Geometry: see drawing. Coordinates: mm, zero at the bounding-box minimum. A direction names the side the tool comes from. Round coordinates to 2 decimals unless told otherwise and drop trailing zeros. Loops run counter-clockwise (first coordinate to the right, second up) from the corner with the lowest first, then second, coordinate; pieces in that order, holes last. Notation, with made-up numbers: (-35.5, 45.5) -> (8.5, 45.5) arc R16 cw to (8.5, 74.5) -> close; hole circle Ø9 at (89, -28.5). An arc over 180 degrees is marked (long way). Write item = value, one per line.
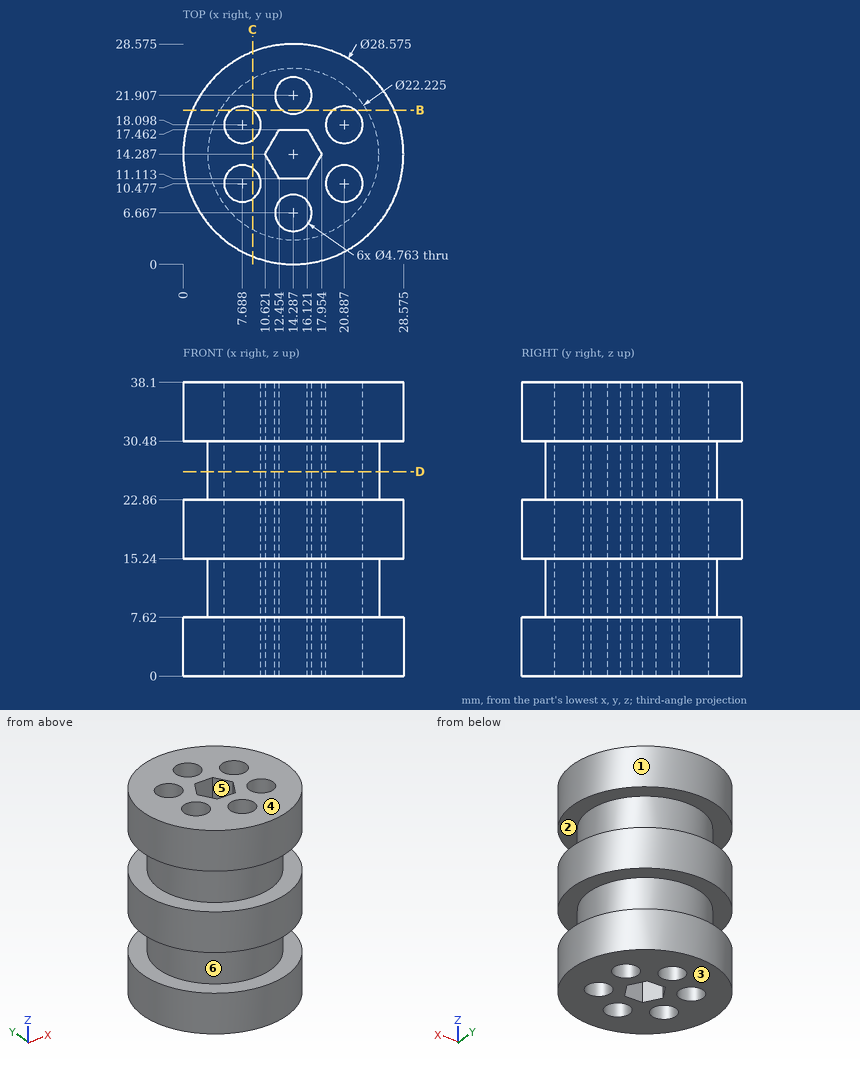
1. Line query: probe 1 along Z at (x, y) = (8.25, 24); probe 2 along Y at (x, z) = (14.25, 18) (1 decimal); probe 3 along X at (y, z) = (8.5, 14) (1 decimal). Output: solid intervals per line, ascending. Write a range as from..to.
Evaluation:
probe_1 = 0..7.62, 15.24..22.86, 30.48..38.1
probe_2 = 0..4.3, 9..11.1, 17.5..19.5, 24.3..28.6
probe_3 = 4.8..6.4, 9..12.8, 15.8..19.6, 22.2..23.8
2. Contact query for flat-ended pins moving along their axis: pin 1 Ø1.5 at (x, z) = (15, 19.5) entering from +Y (1 decimal); pin 2 Ø1.1 at (x, z) = (13.5, 17) entering from -Y; pin 3 Ø4 at (y, z) = (9, 19) entering from -X; pin 4 Ø1.5 at (y, z) = (10, 33) entering from +X. Output: stop coordinate, or through.
Evaluation:
pin_1 = 28.6
pin_2 = 0
pin_3 = 0.38
pin_4 = 28.13
3. Section query D-D (z = 26.5). Return the cut outline in (x, y) (1 decimal).
Evaluation:
outline = circle Ø22.2 at (14.3, 14.3); hole circle Ø4.8 at (7.7, 10.5); hole circle Ø4.8 at (7.7, 18.1); hole (10.6, 14.3) -> (12.5, 11.1) -> (16.1, 11.1) -> (18, 14.3) -> (16.1, 17.5) -> (12.5, 17.5) -> close; hole circle Ø4.8 at (14.3, 6.7); hole circle Ø4.8 at (14.3, 21.9); hole circle Ø4.8 at (20.9, 10.5); hole circle Ø4.8 at (20.9, 18.1)
4. Section query C-C (x = 9). Return the cut outline in (y, z) (1 decimal).
Evaluation:
outline = (1, 0) -> (8.5, 0) -> (8.5, 38.1) -> (1, 38.1) -> (1, 30.5) -> (4.5, 30.5) -> (4.5, 22.9) -> (1, 22.9) -> (1, 15.2) -> (4.5, 15.2) -> (4.5, 7.6) -> (1, 7.6) -> close; (12.5, 0) -> (16.1, 0) -> (16.1, 38.1) -> (12.5, 38.1) -> close; (20.1, 0) -> (27.6, 0) -> (27.6, 7.6) -> (24.1, 7.6) -> (24.1, 15.2) -> (27.6, 15.2) -> (27.6, 22.9) -> (24.1, 22.9) -> (24.1, 30.5) -> (27.6, 30.5) -> (27.6, 38.1) -> (20.1, 38.1) -> close
5. Mould query, pull axis Z, two halves, no side actions, for the marked faces 1, 2 and 3. Classes: released by +Z, released by -Z, zero draft, split by the parting line, or undercut.
Evaluation:
face_1 = zero draft
face_2 = undercut
face_3 = released by -Z
6. Set-up query: the marked faces 4, 5 and 6. Return all of +Z, -Z, +X, -X, +Y, -Y with unobstructed straight access to the full face (end or side cutting, diameter ignored); none if empty.
Evaluation:
face_4 = +Z, +X, -X, +Y, -Y
face_5 = +Z, -Z
face_6 = none
7. Section query B-B (y = 20). Give the number of separate pieces and of enclosed holes in the cut face.
Evaluation:
separate_pieces = 4
enclosed_holes = 0
